from build123d import *

# Parameters (mm, degrees)
F0_W     = 50.8
F0_H     = 469.9
F1_DEPTH = 50.8
F3_DEPTH = 50.801


with BuildPart() as f1:
    # F0 (on Top) → F1 (new body)
    with BuildSketch(Plane.XY):
        with Locations((25.4, 234.95)):
            Rectangle(F0_W, F0_H)
    extrude(amount=F1_DEPTH)

    # F2 (on face) → F3 (cut, through all)
    with BuildSketch(Plane.YZ.offset(50.8)):
        Polygon((0, 50.8), (0, 12.7), (63.5, 50.8), align=None)
        Polygon((406.4, 50.8), (469.9, 12.7), (469.9, 50.8), align=None)
    extrude(amount=-F3_DEPTH, mode=Mode.SUBTRACT)


solid = f1.part
Here's how the part is built. I have some questions about the finished solid (model axes, mm). Round coordinates to 2 decimals unless told otherwise and drop trailing zeros. Order: outer loops, then holes, each group sorted by start corner. A loop starts at its lowest first (then second) coordinate and runs counter-clockwise, first axis right, second up. Notation, with made-up numbers: M 80.5,12.25 L 117.5,12.25 A18 ccw 117.5,37.25 Z; hole C 42,52.25 d1. An arc over 180 degrees is marked long. Return JSON: item names as keys, results as strings. Group by question number.
1. If we section it at C-C on y = 414: List the corners of the cut face in (x, z) for me.
2. If we section it at B-B on x = 28: List the corners of the cut face in (y, z) for me.
3. I'm going to push flat-ended pins straight in: pin 1 Ø6 at (x, z) = (28.5, 17.5) entering from +Y; pin 2 Ø3 at (x, z) = (31, 40.5) entering from +Y; pin 3 Ø12 at (x, z) = (20, 32) entering from -Y; pin 4 Ø10 at (x, y) = (38, 211) entering from -Z. Where does each tip first touch, or does it pass through?
4. Please list where these lines run through material, in increasing order: probe 1 along Y at (x, z) = (37.5, 31); probe 2 along Y at (x, z) = (40.5, 19); probe 3 along Z at (x, y) = (23, 422.5).
5. If we section it at A-A on z = 38.5: List the corners of the cut face in (x, y) for me.
Reply:
{
 "1": {"outline": "M 0,0 L 50.8,0 L 50.8,46.24 L 0,46.24 Z"},
 "2": {"outline": "M 0,0 L 469.9,0 L 469.9,12.7 L 406.4,50.8 L 63.5,50.8 L 0,12.7 Z"},
 "3": {"pin 1": "y = 466.9", "pin 2": "y = 426.07", "pin 3": "y = 22.17", "pin 4": "z = 0"},
 "4": {"probe 1": "30.5 to 439.4", "probe 2": "10.5 to 459.4", "probe 3": "0 to 41.14"},
 "5": {"outline": "M 0,43 L 50.8,43 L 50.8,426.9 L 0,426.9 Z"}
}
